Part model, mm, in its own coordinate system. Face numbers are marked on the shaded views. A direction names the side the tool comes from. Round coordinates to 2 decimals unless told otherwise and drop trailing zeros. Loops run counter-clockwise (first coordinate to the right, second up) from the corner with the lowest first, then second, coordinate; pieces in that order, holes last.
1) Band-saw the part on A-A, the plane y = 1.75. Write the cut outline in (x, z).
2) Band-saw the part on B-B, the plane z = -2.75. Write the cut outline in (x, y).
3) Drop flat-ended pins along their axis: P1, Ø0.6, axis at x = 3.5, z = -2, coming from the +Y side; P2, Ø0.6, axis at x = 1, z = -4.5, coming from the +Y side. Give the stop position or say it passes through.
4) Band-saw the part on C-C, the plane x = 6.5. Write the cut outline in (y, z).
5) Band-saw the part on D-D, the plane x = 2.75. Write the cut outline in (y, z), then the cut area to 3 significant figures.
6) 3-axis set-ups, long thin cutter, end or side, ignore diameter. For the marked faces 1 and 2: which of +Z, -Z, +X, -X, +Y, -Y reach the whole face in a straight line?
7) Probe line 1 (Y direction, x = 5.25, z = 2); line 2 (Y direction, x = 8.25, z = -3.25). List the from-to ranges inside material, lowest first.
from build123d import *

# Parameters (mm, degrees)
BOSS_EXTRUDE1_DEPTH      = 5
BOSS_EXTRUDE1_DEPTH_BACK = 9
SKETCH1_W                = 10
SKETCH1_H                = 2
CUT_EXTRUDE1_DEPTH       = 18
LPATTERN2_COUNT          = 6
LPATTERN2_PITCH          = 1.4


with BuildPart() as part:
    # Sketch1 → Boss-Extrude1 (new, two sides: drawn at the far end of the back side and taken through both)
    with BuildSketch(Plane.XY.offset(-BOSS_EXTRUDE1_DEPTH_BACK)):
        with Locations((5, 1)):
            Rectangle(SKETCH1_W, SKETCH1_H)
    extrude(amount=BOSS_EXTRUDE1_DEPTH + BOSS_EXTRUDE1_DEPTH_BACK)

    # Sketch3 → Cut-Extrude1 (cut)
    with BuildSketch(Plane.XY.offset(5)):
        Polygon((0.689824634, 1), (1.189824634, 1), (1.619628875, 2.012555339), (0.260020392, 2.012555339), align=None)
    cut_extrude1 = extrude(amount=-CUT_EXTRUDE1_DEPTH, mode=Mode.SUBTRACT)

    # LPattern2: Cut-Extrude1 ×6
    with Locations(*[(i * LPATTERN2_PITCH, 0, 0) for i in range(1, LPATTERN2_COUNT)]):
        add(cut_extrude1, mode=Mode.SUBTRACT)


solid = part.part
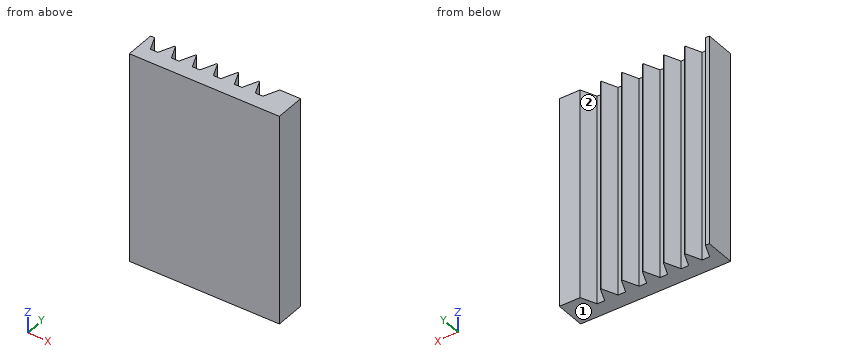
Reported:
1. outline: (0, -9) - (0.37, -9) - (0.37, 5) - (0, 5) - close; (1.51, -9) - (1.77, -9) - (1.77, 5) - (1.51, 5) - close; (2.91, -9) - (3.17, -9) - (3.17, 5) - (2.91, 5) - close; (4.31, -9) - (4.57, -9) - (4.57, 5) - (4.31, 5) - close; (5.71, -9) - (5.97, -9) - (5.97, 5) - (5.71, 5) - close; (7.11, -9) - (7.37, -9) - (7.37, 5) - (7.11, 5) - close; (8.51, -9) - (10, -9) - (10, 5) - (8.51, 5) - close
2. outline: (0, 0) - (10, 0) - (10, 2) - (8.61, 2) - (8.19, 1) - (7.69, 1) - (7.27, 2) - (7.21, 2) - (6.79, 1) - (6.29, 1) - (5.87, 2) - (5.81, 2) - (5.39, 1) - (4.89, 1) - (4.47, 2) - (4.41, 2) - (3.99, 1) - (3.49, 1) - (3.07, 2) - (3.01, 2) - (2.59, 1) - (2.09, 1) - (1.67, 2) - (1.61, 2) - (1.19, 1) - (0.69, 1) - (0.27, 2) - (0, 2) - close
3. P1: stops at y = 1.68
3. P2: stops at y = 1.26
4. outline: (0, -9) - (1, -9) - (1, 5) - (0, 5) - close
5. outline: (0, -9) - (1.38, -9) - (1.38, 5) - (0, 5) - close
5. area: 19.3 mm2
6. face 1: -Z, +X, -X, +Y, -Y
6. face 2: +Z, -Z, +Y
7. line 1: y = 0 to 1
7. line 2: y = 0 to 1.14
